from build123d import *

# Parameters (mm, degrees)
SKETCH_1_R      = 8
SKETCH_1_R_2    = 2
EXTRUDE_1_DEPTH = 5


with BuildPart() as part:
    # 草图1 → 凸台-拉伸1 (new body)
    with BuildSketch(Plane.XY):
        with BuildLine():
            Line((0.397515528, -15.995061157), (161.298136646, -11.996295867))
            ThreePointArc((161.298136646, -11.996295867), (173, 0), (161.298136646, 11.996295867))
            Line((161.298136646, 11.996295867), (0.397515528, 15.995061157))
            ThreePointArc((0.397515528, 15.995061157), (-16, 0), (0.397515528, -15.995061157))
        make_face()
        Circle(SKETCH_1_R, mode=Mode.SUBTRACT)
        with Locations((161, 0)):
            Circle(SKETCH_1_R_2, mode=Mode.SUBTRACT)
        with Locations((64.4, 0)):
            Circle(SKETCH_1_R_2, mode=Mode.SUBTRACT)
        with BuildLine():
            Line((18.4, 4), (54.4, 4))
            ThreePointArc((54.4, 4), (58.4, 0), (54.4, -4))
            Line((54.4, -4), (18.4, -4))
            ThreePointArc((18.4, -4), (14.4, 0), (18.4, 4))
        make_face(mode=Mode.SUBTRACT)
        with BuildLine():
            Line((75, 4), (153, 4))
            ThreePointArc((153, 4), (157, 0), (153, -4))
            Line((153, -4), (75, -4))
            ThreePointArc((75, -4), (71, 0), (75, 4))
        make_face(mode=Mode.SUBTRACT)
    extrude(amount=EXTRUDE_1_DEPTH)


solid = part.part
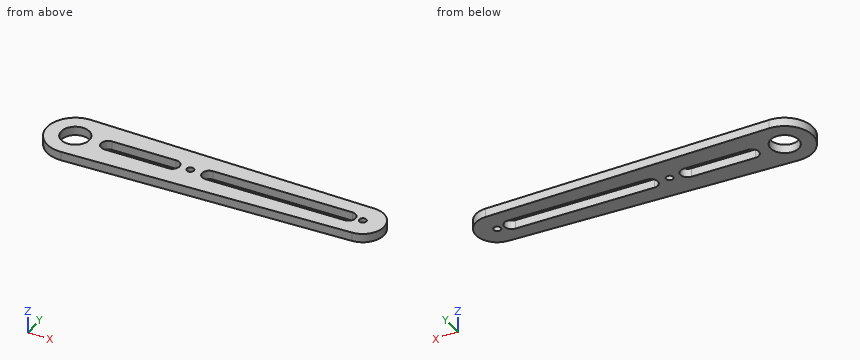
Input: part model. Units: mm. Frame: model coordinates. Coordinates: 2 decimals unless noted, no trailing zeros. Loops run counter-clockwise (first coordinate to the right, second up) from the corner with the lowest first, then second, coordinate; pieces in that order, holes last. Notation, with made-up numbers: (-36, -12.5) - (-10, -12.5) arc R20 cw to (-10, 5.5) - close; hole circle Ø1 at (-10.5, 24). An arc over 180 degrees is marked (long way). Answer in a Markdown table with one row per item. Add a question column.
Item 1: Section query C-C on x = 35.5. Return the cut outline in (y, z), then the cut area to 3 significant figures.
Item 2: Line query: line 1 along Y through (x, z) = (161, 1.95); line 2 along Y through (x, z) = (0, 1.8); line 3 along X through (y, z) = (6.5, 2.45). Output: solid intervals per line, ascending. Write a range as [from, to].
Item 3: Contact query for flat-ended pins moving along their axis: P1, Ø1.5, axis at x = 37.5, z = 3, coming from the +Y side; P2, Ø1.5, axis at x = 93, z = 0.5, coming from the -Y side; P3, Ø2.5, axis at x = 100.5, z = 3.5, coming from the -Y side. Output: stop coordinate, or through.
Item 4: Section query B-B on x = 64.4. Return the cut outline in (y, z).
Item 5: Section query D-D on y = 10. Return the cut outline in (x, z).
Item 6: Section query A-A on z = 2.15. Return the cut outline in (x, y).
Recorded:
| question | item | result |
|---|---|---|
| 1 | outline | (-15.12, 0) - (-4, 0) - (-4, 5) - (-15.12, 5) - close; (4, 0) - (15.12, 0) - (15.12, 5) - (4, 5) - close |
| 1 | area | 111 mm^2 |
| 2 | line 1 | [-12, -2], [2, 12] |
| 2 | line 2 | [-16, -8], [8, 16] |
| 2 | line 3 | [-14.62, -4.66], [4.66, 171.09] |
| 3 | P1 | y = 15.09 |
| 3 | P2 | y = -13.71 |
| 3 | P3 | y = -13.54 |
| 4 | outline | (-14.4, 0) - (-2, 0) - (-2, 5) - (-14.4, 5) - close; (2, 0) - (14.4, 0) - (14.4, 5) - (2, 5) - close |
| 5 | outline | (-12.49, 0) - (167.63, 0) - (167.63, 5) - (-12.49, 5) - close |
| 6 | outline | (0.4, -16) - (161.3, -12) arc R12 ccw to (161.3, 12) - (0.4, 16) arc R16 ccw (long way) to start; hole circle Ø16 at (0, 0); hole (18.4, -4) - (54.4, -4) arc R4 ccw to (54.4, 4) - (18.4, 4) arc R4 ccw to start; hole circle Ø4 at (64.4, 0); hole (75, -4) - (153, -4) arc R4 ccw to (153, 4) - (75, 4) arc R4 ccw to start; hole circle Ø4 at (161, 0) |
